Could you check a few things on this model? Use its own coordinates, in mm. Face numbers are marked on the shaded views. A direction names the side the tool comes from. Give positions to 0.01 mm unless a question says otherwise; leave off trailing zeros. Write each loop counter-clockwise with the first axis right and the second up, starting at its lowest first coordinate (ties: lowest second). Pieces come first, ordered by that corner, then holes. Notation, with made-up numbers: (-6.75, 43.25) -> (20.25, 43.25) arc R34 ccw to (20.25, 80.25) -> close; hole circle Ø7 at (75, -12.5). An arc over 180 degrees is marked (long way). Write item = value, one per line. Start each with the question number.
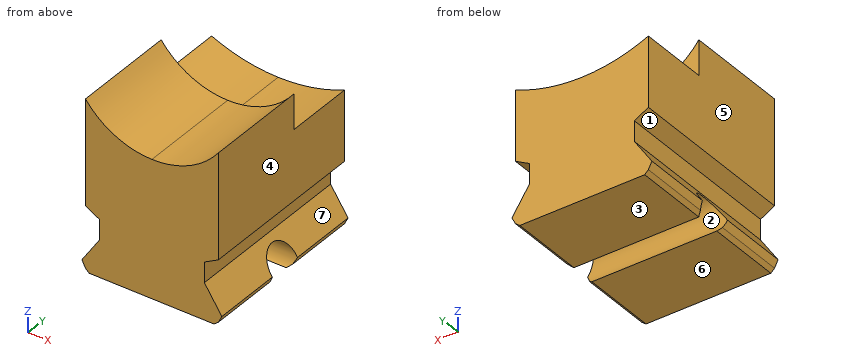
```python
from build123d import *

# Parameters (mm, degrees)
F1_DEPTH       = 25
F3_DEPTH       = 25
F5_DEPTH       = 10
F6_DEPTH       = 5
F8_DEPTH       = 25
F10_DEPTH      = 25
F10_DEPTH_BACK = 25


with BuildPart() as f1:
    # F0 (on Front) → F1 (new body)
    with BuildSketch(Plane.XZ):
        with BuildLine():
            ThreePointArc((8.0529790092, -2), (3.1988570495, -1.4945793088), (-1.4470209908, 0))
            Line((-1.4470209908, 0), (-1.4470209908, -17))
            Line((-1.4470209908, -17), (17.5529790092, -17))
            Line((17.5529790092, -17), (17.5529790092, 0))
            ThreePointArc((17.5529790092, 0), (12.907100969, -1.4945793088), (8.0529790092, -2))
        make_face()
        Polygon((17.5529790092, -17), (-1.4470209908, -17), (-1.9470209908, -17.75), (18.0529790092, -17.75), align=None)
        Polygon((18.0529790092, -17.75), (-1.9470209908, -17.75), (-1.4470209908, -18.75), (17.5529790092, -18.75), align=None)
        Polygon((17.5529790092, -18.75), (-1.4470209908, -18.75), (-0.9180161287, -19.25), (16.9282071292, -19.25), align=None)
        with BuildLine():
            Line((8.0529790092, 0), (-1.4470209908, 0))
            ThreePointArc((-1.4470209908, 0), (3.1988570495, -1.4945793088), (8.0529790092, -2))
            Line((8.0529790092, -2), (8.0529790092, 0))
        make_face()
        with BuildLine():
            Line((17.5529790092, 0), (8.0529790092, 0))
            Line((8.0529790092, 0), (8.0529790092, -2))
            ThreePointArc((8.0529790092, -2), (12.907100969, -1.4945793088), (17.5529790092, 0))
        make_face()
    extrude(amount=F1_DEPTH)

    # F2 (on face) → F3 (cut)
    with BuildSketch(Plane.XZ.offset(25)):
        Polygon((-1.4470209908, -14), (-1.4470209908, -17), (0.5529790092, -14), (0.5529790092, -11.1042056233), (-1.4470209908, -11.1042056233), align=None)
        Polygon((-1.4470209908, -10), (-1.4470209908, -11.1042056233), (0.5529790092, -11.1042056233), align=None)
        Polygon((17.5529790092, -10), (15.5529790092, -11.1042056233), (15.5529790092, -14), (17.5529790092, -17), align=None)
    extrude(amount=-F3_DEPTH, mode=Mode.SUBTRACT)

    # F4 (on face) → F5 (cut)
    with BuildSketch(Plane(origin=(0, 0, 0), x_dir=(-1, 0, 0), z_dir=(0, 1, 0))):
        with BuildLine():
            Line((-8.0529790092, -2), (-8.0529790092, 0))
            Line((-8.0529790092, 0), (-17.5529790092, 0))
            ThreePointArc((-17.5529790092, 0), (-12.907100969, -1.4945793088), (-8.0529790092, -2))
        make_face()
        with BuildLine():
            Line((1.4470209908, 0), (-8.0529790092, 0))
            Line((-8.0529790092, 0), (-8.0529790092, -2))
            ThreePointArc((-8.0529790092, -2), (-3.1988570495, -1.4945793088), (1.4470209908, 0))
        make_face()
    extrude(amount=-F5_DEPTH, mode=Mode.SUBTRACT)

    # F6 (add): a face of the model
    f6_faces = [f1.faces().sort_by_distance(p)[0] for p in [
        (8.0529790092, -17.5, 0),
    ]]
    extrude(f6_faces, amount=F6_DEPTH)

    # F7 (on face) → F8 (cut)
    with BuildSketch(Plane.XZ.offset(25)):
        with BuildLine():
            Line((17.5529790092, 5), (-1.4470209908, 5))
            ThreePointArc((-1.4470209908, 5), (2.7534507283, 1.5392513471), (8.0529790092, 0.3))
            ThreePointArc((8.0529790092, 0.3), (13.3525072901, 1.5392513471), (17.5529790092, 5))
        make_face()
    extrude(amount=-F8_DEPTH, mode=Mode.SUBTRACT)

    # F9 (on face) → F10 (cut, two sides)
    with BuildSketch(Plane.YZ.offset(17.5529790092)) as f10_sk:
        with BuildLine():
            Line((-15, -17.5), (-10, -17.5))
            ThreePointArc((-10, -17.5), (-12.5, -15), (-15, -17.5))
        make_face()
        with BuildLine():
            ThreePointArc((-15, -17.5), (-12.5, -20), (-10, -17.5))
            Line((-10, -17.5), (-15, -17.5))
        make_face()
    extrude(amount=-F10_DEPTH, mode=Mode.SUBTRACT)
    extrude(f10_sk.sketch, amount=F10_DEPTH_BACK, mode=Mode.SUBTRACT)


solid = f1.part
```
(1) We'd pull the mould along Z, two halves only. Please class the marked faces 1, 2, 3 and 4: released by +Z, released by -Z, zero draft, split by the parting line, or undercut.
(2) On a 3-axis mill with a long thin cutter (end or side, diameter ignored), from which of +Z, -Z, +X, -X, +Y, -Y can I reach the whole of each face in a straight line? I mean the marked faces 5, 6 and 7. Say none if no direction works.
(3) Imagine slicing it at B-B (y = -22.75). Please give me the cut outline in (x, z).
(4) Imagine slicing it at A-A (z = 2). Please give me the cut outline in (x, y), then the cut area to 3 significant figures.
(5) I'm going to push flat-ended pins straight in: pin 1 (1.5 mm diameter, centred on x = 8.5, y = -16, fed in from +Z); pin 2 (2.5 mm diameter, centred on y = -11, z = -12.5, fed in from -X); pin 3 (6 mm diameter, centred on y = -16, z = -3.5, fed in from -X). Where does each tip first touch, or does it pass through?
(6) If I drill on line 1 along Y through (x, z) = (5.25, -15.75); line 2 along Y through (x, z) = (13.5, -17.5); line 3 along X through (y, z) = (-8.5, -4.25), over which ranges is the centre line in solid material (lowest first)? Write a range as from..to.
(7) Imagine slicing it at C-C (x = 4). Please give me the cut outline in (y, z), then the cut area to 3 significant figures.
(8) Imagine slicing it at D-D (z = -4.75). Please give me the cut outline in (x, y).
Answers below:
q1.face_1 = undercut
q1.face_2 = undercut
q1.face_3 = released by -Z
q1.face_4 = zero draft
q2.face_5 = +Z, -X, +Y, -Y
q2.face_6 = -Z, +X, -X, +Y, -Y
q2.face_7 = +X, +Y, -Y
q3.outline = (-1.95, -17.75) -> (-1.45, -18.75) -> (-0.92, -19.25) -> (16.93, -19.25) -> (17.55, -18.75) -> (18.05, -17.75) -> (15.55, -14) -> (15.55, -11.1) -> (17.55, -10) -> (17.55, 5) arc R11.95 cw to (-1.45, 5) -> (-1.45, -10) -> (0.55, -11.1) -> (0.55, -14) -> close
q4.outline = (-1.45, -25) -> (1.91, -25) -> (1.91, -10) -> (-1.45, -10) -> close; (14.2, -25) -> (17.55, -25) -> (17.55, -10) -> (14.2, -10) -> close
q4.area = 101 mm^2
q5.pin_1 = 0.36
q5.pin_2 = 0.55
q5.pin_3 = -1.45
q6.line_1 = -25..-14.29, -10.71..0
q6.line_2 = -25..-15, -10..0
q6.line_3 = -1.45..17.55
q7.outline = (-25, -19.25) -> (-14.29, -19.25) arc R2.5 cw (long way) to (-10.71, -19.25) -> (0, -19.25) -> (0, -1.65) -> (-10, -1.65) -> (-10, 1.01) -> (-25, 1.01) -> close
q7.area = 462 mm^2
q8.outline = (-1.45, -25) -> (17.55, -25) -> (17.55, 0) -> (-1.45, 0) -> close
